from build123d import *

# Parameters (mm, degrees)
F0_W     = 19.05
F0_H     = 19.05
F1_DEPTH = 57.15
F2_W     = 19.05
F2_H     = 38.1
F3_DEPTH = 19.05
F4_W     = 18.542
F4_H     = 19.05
F5_DEPTH = 19.05


# Not quite as in the source:
# - a feature names something its author has since deleted; it is built from what else it names


with BuildPart() as f1:
    # F0 (on Top) → F1 (new body)
    with BuildSketch(Plane.XY):
        with Locations((9.525, -9.525)):
            Rectangle(F0_W, F0_H)
    extrude(amount=F1_DEPTH)

    # F2 (on face) → F3 (join)
    with BuildSketch(Plane.XZ.offset(19.05)):
        with Locations((9.525, 38.1)):
            Rectangle(F2_W, F2_H)
    extrude(amount=F3_DEPTH)

    # F4 (on face) → F5 (join)
    with BuildSketch(Plane.YZ.offset(19.05)):
        with Locations((-28.829, 28.575)):
            Rectangle(F4_W, F4_H)
    extrude(amount=F5_DEPTH)


solid = f1.part
Part model, mm, in its own coordinate system. A direction names the side the tool comes from. Round coordinates to 2 decimals unless told otherwise and drop trailing zeros. Write each loop counter-clockwise with the first axis right and the second up, starting at its lowest first coordinate (ties: lowest second). Pieces come first, ordered by that corner, then holes. Notation, with made-up numbers: M 45.25,51.5 L 87.25,51.5 A31 cw 87.25,89.5 Z; hole C 3,-16.75 d10. An arc over 180 degrees is marked long. Return JSON: item names as keys, results as strings. Group by question number.
(1) Pin check, flat tips, straight feed: pin 1 Ø15 at (x, y) = (33, -26) entering from +Z; pin 2 Ø15 at (x, z) = (32, 31.5) entering from +Y; pin 3 Ø3 at (x, z) = (17, 16.5) entering from -Y. Stop position of each tip, or through.
(2) Which spindle directions (+Z, -Z, +X, -X, +Y, -Y) get a long thin tool onto all of the face, cutting with end or side? Do faces 1 (the face through (19, -29, 19.05)), 2 (the face through (28, -19.558, 28)), 3 (the face through (28, -29, 38.1)). Say none if no direction does.
(3) Saw through at B-B on z = 28.5. Write the cut outline in (x, y).
(4) Saw through at D-D on z = 10.5. Write the cut outline in (x, y).
(5) Saw through at C-C on x = 26. Write the cut outline in (y, z).
(6) Drill centre lines: probe 1 along X at (y, z) = (-34, 40.5); probe 2 along Z at (x, y) = (15, -23); probe 3 along Y at (x, z) = (28.5, 20.5). Where is each one in solid material? Low to high.
(7) Saw through at A-A on y = -31.5. Write the cut outline in (x, z).
Returned:
{
 "1": {"pin 1": "z = 38.1", "pin 2": "y = -19.56", "pin 3": "y = -19.05"},
 "2": {"face 1": "-Z, +X, -X, -Y", "face 2": "+Z, -Z, +X, +Y", "face 3": "+Z, +X, +Y, -Y"},
 "3": {"outline": "M 0,-38.1 L 38.1,-38.1 L 38.1,-19.56 L 19.05,-19.56 L 19.05,0 L 0,0 Z"},
 "4": {"outline": "M 0,-19.05 L 19.05,-19.05 L 19.05,0 L 0,0 Z"},
 "5": {"outline": "M -38.1,19.05 L -19.56,19.05 L -19.56,38.1 L -38.1,38.1 Z"},
 "6": {"probe 1": "0 to 19.05", "probe 2": "19.05 to 57.15", "probe 3": "-38.1 to -19.56"},
 "7": {"outline": "M 0,19.05 L 38.1,19.05 L 38.1,38.1 L 19.05,38.1 L 19.05,57.15 L 0,57.15 Z"}
}
